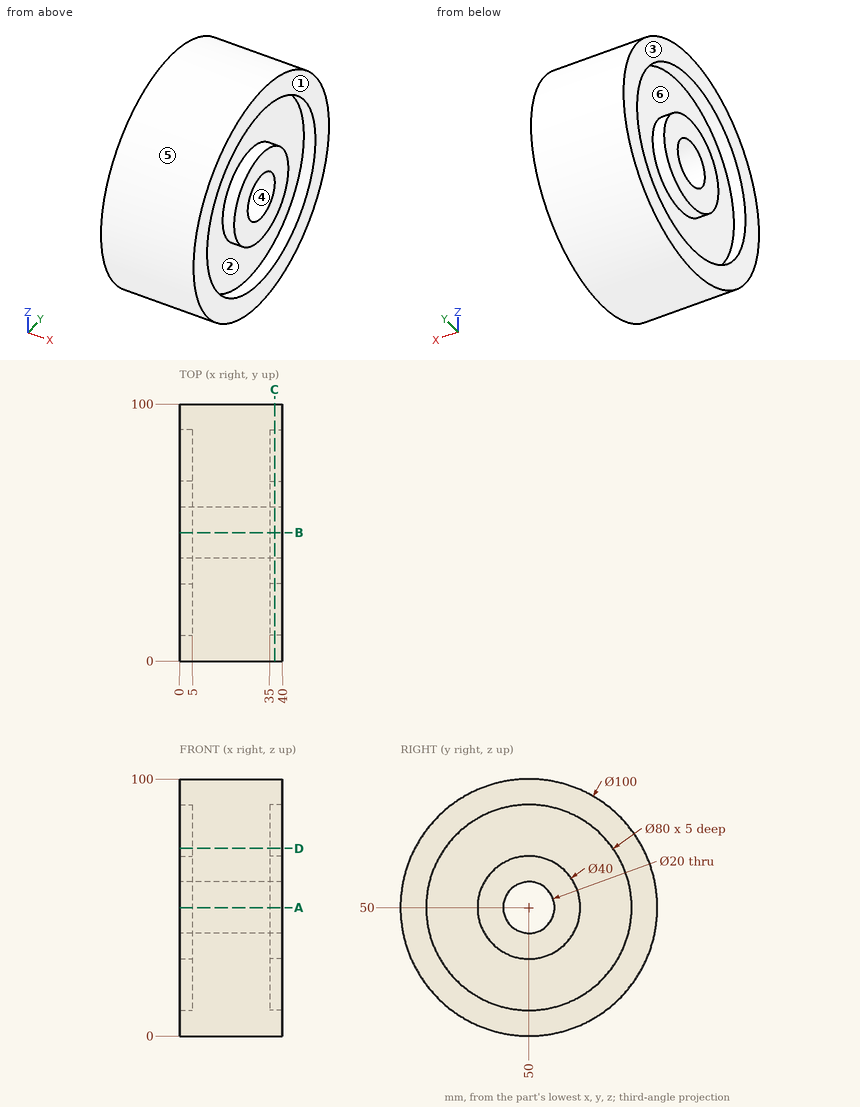
Design review of the part shown in the three views and the two pictorial views. Dimensions are in mm from the part's minimum x, y and z. A direction names the side the tool comes from. Give positions to 0.01 mm unless a question says otherwise; leave off trailing zeros. Loops run counter-clockwise (first coordinate to the right, second up) from the corner with the lowest first, then second, coordinate; pieces in that order, holes last. Notation, with made-up numbers: M 70,-36.75 L 112,-36.75 A6 ccw 112,-26.75 Z; hole C 14,45 d7. An arc over 180 degrees is marked long. Write item = value, one per line.
Q1. We need section A-A (z = 50). Give the boundary of the cut face in (x, y).
Output values:
outline = M 0,0 L 40,0 L 40,10 L 35,10 L 35,30 L 40,30 L 40,40 L 0,40 L 0,30 L 5,30 L 5,10 L 0,10 Z; M 0,60 L 40,60 L 40,70 L 35,70 L 35,90 L 40,90 L 40,100 L 0,100 L 0,90 L 5,90 L 5,70 L 0,70 Z
Q2. For the marked faces 1 and 2, list the 3-axis set-ups (+Z, -Z, +X, -X, +Y, -Y) from which the entire face can be reached by the end or side of a thin tool; tool diameter is ignored.
Output values:
face_1 = +Z, -Z, +X, +Y, -Y
face_2 = +X
Q3. We need section C-C (x = 37). Give the boundary of the cut face in (y, z), plus the area to 3 significant figures.
Output values:
outline = C 50,50 d100; C 50,50 d40; hole C 50,50 d80; hole C 50,50 d20
area = 3,770 mm^2
Q4. Insertion check: pin 1 (8 mm diameter, centred on x = 23.5, z = 81.5, fed in from +Y); pin 2 (5 mm diameter, centred on x = 16, y = 63, fed in from -Z); pin 3 (10 mm diameter, centred on y = 71.5, z = 32.5, fed in from +X). Each pin has a flat end and moves straight along its axis. Give the tip position at first contact, or say it passes through.
Output values:
pin_1 = 91.76
pin_2 = 1.11
pin_3 = 35
Q5. We need section D-D (z = 73). Give the boundary of the cut face in (x, y), plus the area to 3 significant figures.
Output values:
outline = M 0,5.6 L 40,5.6 L 40,17.27 L 35,17.27 L 35,82.73 L 40,82.73 L 40,94.4 L 0,94.4 L 0,82.73 L 5,82.73 L 5,17.27 L 0,17.27 Z
area = 2,900 mm^2
Q6. Draft analysis for pull direction Y (two halves, no side actions). For the marked faces 3, 4, 5 and 6, state which applies: +Y half, -Y half, draft (parallel to the pull), parting line (faces both ways), or undercut.
Output values:
face_3 = draft
face_4 = undercut
face_5 = parting line
face_6 = undercut
Q7. To check wall thickness, follow line 1 (Z direction, x = 3.2, y = 50); line 2 (Z direction, x = 10, y = 50); line 3 (Y direction, x = 3, z = 33.5). State the ranges of each line that lie inside material, in increasing order. Write a range as [from, to].
Output values:
line_1 = [0, 10], [30, 40], [60, 70], [90, 100]
line_2 = [0, 40], [60, 100]
line_3 = [2.8, 13.56], [38.7, 61.3], [86.44, 97.2]
